Input: part model. Units: mm. Frame: model coordinates. Round coordinates to 2 decimals unless told otherwise and drop trailing zeros. Order: outer loops, then holes, each group sorted by start corner. A loop starts at its lowest first (then second) coordinate and runs counter-clockwise, first axis right, second up. Notation, with made-up numbers: (18.5, 57.25) - (29.5, 57.25) arc R32 ccw to (29.5, 95.25) - close; hole circle Ø1 at (26.5, 3). An arc over 180 degrees is marked (long way). One line per item, written item: value. Start each with the question number.
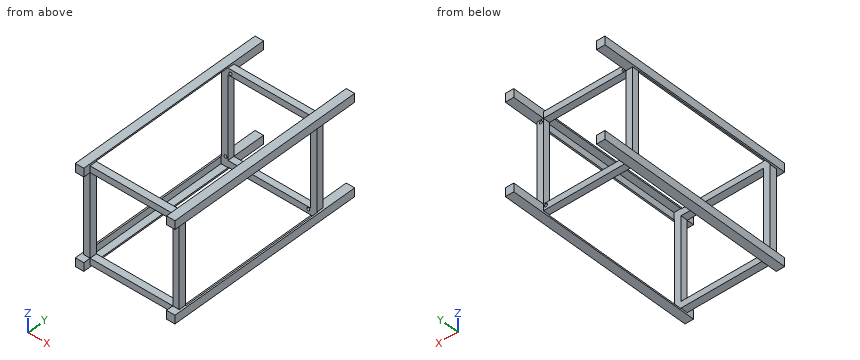
from build123d import *

# Parameters (mm, degrees)
SKETCH1_W           = 100
SKETCH1_H           = 100
BOSS_EXTRUDE1_DEPTH = 200
SKETCH2_W           = 83
SKETCH2_H           = 83
CUT_EXTRUDE1_DEPTH  = 200
SKETCH3_W           = 83
SKETCH3_H           = 14
SKETCH3_H_2         = 146.5
SKETCH3_H_3         = 66
CUT_EXTRUDE2_DEPTH  = 200
SKETCH4_W           = 83
SKETCH4_H           = 14
SKETCH4_H_2         = 146.5
SKETCH4_H_3         = 66
CUT_EXTRUDE3_DEPTH  = 200
SKETCH5_W           = 83
SKETCH5_H           = 4
SKETCH5_W_2         = 4
SKETCH5_H_2         = 83
CUT_EXTRUDE4_DEPTH  = 200
SKETCH8_W           = 97
SKETCH8_H           = 97
CUT_EXTRUDE5_DEPTH  = 146.5
CUT_EXTRUDE6_REACH  = 220.836
SKETCH9_R           = 1.5


with BuildPart() as part:
    # Sketch1 → Boss-Extrude1 (new body)
    with BuildSketch(Plane(origin=(0, 0, 0), x_dir=(1, 0, 0), z_dir=(0, 1, 0))):
        with Locations((50, 50)):
            Rectangle(SKETCH1_W, SKETCH1_H)
    extrude(amount=BOSS_EXTRUDE1_DEPTH)

    # Sketch2 → Cut-Extrude1 (cut)
    with BuildSketch(Plane(origin=(0, 200, 0), x_dir=(1, 0, 0), z_dir=(0, 1, 0))):
        with Locations((50, 50)):
            Rectangle(SKETCH2_W, SKETCH2_H)
    extrude(amount=-CUT_EXTRUDE1_DEPTH, mode=Mode.SUBTRACT)

    # Sketch3 → Cut-Extrude2 (cut)
    with BuildSketch(Plane.XY):
        with Locations((50, 0)):
            Rectangle(SKETCH3_W, SKETCH3_H)
        with Locations((50, 87.25)):
            Rectangle(SKETCH3_W, SKETCH3_H_2)
        with Locations((50, 200)):
            Rectangle(SKETCH3_W, SKETCH3_H_3)
    extrude(amount=-CUT_EXTRUDE2_DEPTH, mode=Mode.SUBTRACT)

    # Sketch4 → Cut-Extrude3 (cut)
    with BuildSketch(Plane.ZY):
        with Locations((-50, 0)):
            Rectangle(SKETCH4_W, SKETCH4_H)
        with Locations((-50, 87.25)):
            Rectangle(SKETCH4_W, SKETCH4_H_2)
        with Locations((-50, 200)):
            Rectangle(SKETCH4_W, SKETCH4_H_3)
    extrude(amount=-CUT_EXTRUDE3_DEPTH, mode=Mode.SUBTRACT)

    # Sketch5 → Cut-Extrude4 (cut)
    with BuildSketch(Plane.XZ.offset(-7)):
        with Locations((50, 0)):
            Rectangle(SKETCH5_W, SKETCH5_H)
        with Locations((100, -50)):
            Rectangle(SKETCH5_W_2, SKETCH5_H_2)
        with Locations((50, -100)):
            Rectangle(SKETCH5_W, SKETCH5_H)
        with Locations((0, -50)):
            Rectangle(SKETCH5_W_2, SKETCH5_H_2)
    extrude(amount=-CUT_EXTRUDE4_DEPTH, mode=Mode.SUBTRACT)

    # Sketch8 → Cut-Extrude5 (cut)
    with BuildSketch(Plane.XZ.offset(-160.5)):
        with Locations((50, -50)):
            Rectangle(SKETCH8_W, SKETCH8_H)
    extrude(amount=CUT_EXTRUDE5_DEPTH, mode=Mode.SUBTRACT)

    # Sketch9 → Cut-Extrude6 (cut, up to next)
    with BuildSketch(Plane(origin=(0, 167, 0), x_dir=(1, 0, 0), z_dir=(0, 1, 0)), mode=Mode.PRIVATE) as cut_extrude6_sk1:
        with Locations(Location((6, 89, 0), (0, 0, 270))):
            Circle(SKETCH9_R)
    cut_extrude6_tool1 = extrude(cut_extrude6_sk1.sketch, amount=-CUT_EXTRUDE6_REACH, mode=Mode.PRIVATE) & part.part
    # Sketch9 → Cut-Extrude6 (cut, up to next)
    with BuildSketch(Plane(origin=(0, 167, 0), x_dir=(1, 0, 0), z_dir=(0, 1, 0)), mode=Mode.PRIVATE) as cut_extrude6_sk2:
        with Locations(Location((89, 94, 0), (0, 0, 270))):
            Circle(SKETCH9_R)
    cut_extrude6_tool2 = extrude(cut_extrude6_sk2.sketch, amount=-CUT_EXTRUDE6_REACH, mode=Mode.PRIVATE) & part.part
    # Sketch9 → Cut-Extrude6 (cut, up to next)
    with BuildSketch(Plane(origin=(0, 167, 0), x_dir=(1, 0, 0), z_dir=(0, 1, 0)), mode=Mode.PRIVATE) as cut_extrude6_sk3:
        with Locations(Location((94, 11, 0), (0, 0, 270))):
            Circle(SKETCH9_R)
    cut_extrude6_tool3 = extrude(cut_extrude6_sk3.sketch, amount=-CUT_EXTRUDE6_REACH, mode=Mode.PRIVATE) & part.part
    # Sketch9 → Cut-Extrude6 (cut, up to next)
    with BuildSketch(Plane(origin=(0, 167, 0), x_dir=(1, 0, 0), z_dir=(0, 1, 0)), mode=Mode.PRIVATE) as cut_extrude6_sk4:
        with Locations(Location((11, 6, 0), (0, 0, 270))):
            Circle(SKETCH9_R)
    cut_extrude6_tool4 = extrude(cut_extrude6_sk4.sketch, amount=-CUT_EXTRUDE6_REACH, mode=Mode.PRIVATE) & part.part
    add(cut_extrude6_tool1.solids().sort_by_distance((6, 167, -89))[0], mode=Mode.SUBTRACT)
    add(cut_extrude6_tool2.solids().sort_by_distance((89, 167, -94))[0], mode=Mode.SUBTRACT)
    add(cut_extrude6_tool3.solids().sort_by_distance((94, 167, -11))[0], mode=Mode.SUBTRACT)
    add(cut_extrude6_tool4.solids().sort_by_distance((11, 167, -6))[0], mode=Mode.SUBTRACT)


solid = part.part
1. Section B-B (z = -31). Return the cut outline in (x, y), then the cut area to 4 significant figures.
2. Section C-C (x = 65.5). Return the cut outline in (y, z), then the cut area to 4 significant figures.
3. Section A-A (y = 64). Return the cut outline in (x, z), then the cut area to 3 significant figures.
4. Line query: line 1 (X direction, y = 165, z = -11); line 2 (X direction, y = 165, z = -89); line 3 (X direction, y = 162, z = -6). Output: solid intervals per line, ascending. Write a range as from..to.
5. Pin query (flat end, axial travel): pin 1 (7.5 mm diameter, centred on x = 60, y = 10, fed in from +Z); pin 2 (3.5 mm diameter, centred on y = 9.5, z = -58, fed in from -X); pin 3 (5 mm diameter, centred on x = 94.5, z = -48, fed in from +Y). Return the tip coordinate at first contact, or that it passes through.
Solved:
1. outline: (2, 7) - (8.5, 7) - (8.5, 14) - (2, 14) - close; (2, 160.5) - (8.5, 160.5) - (8.5, 167) - (2, 167) - close; (91.5, 7) - (98, 7) - (98, 14) - (91.5, 14) - close; (91.5, 160.5) - (98, 160.5) - (98, 167) - (91.5, 167) - close
1. area: 175.5 mm²
2. outline: (7, -98) - (14, -98) - (14, -91.5) - (7, -91.5) - close; (7, -8.5) - (14, -8.5) - (14, -2) - (7, -2) - close; (160.5, -98) - (167, -98) - (167, -91.5) - (160.5, -91.5) - close; (160.5, -8.5) - (167, -8.5) - (167, -2) - (160.5, -2) - close
2. area: 175.5 mm²
3. outline: (0, -100) - (8.5, -100) - (8.5, -98.5) - (1.5, -98.5) - (1.5, -91.5) - (0, -91.5) - close; (0, -8.5) - (1.5, -8.5) - (1.5, -1.5) - (8.5, -1.5) - (8.5, 0) - (0, 0) - close; (91.5, -100) - (100, -100) - (100, -91.5) - (98.5, -91.5) - (98.5, -98.5) - (91.5, -98.5) - close; (91.5, -1.5) - (98.5, -1.5) - (98.5, -8.5) - (100, -8.5) - (100, 0) - (91.5, 0) - close
3. area: 93.0 mm²
4. line 1: x = 2..8.5, 91.5..92.5, 95.5..98
4. line 2: x = 2..4.5, 7.5..8.5, 91.5..98
4. line 3: x = 0..9.5, 12.5..100
5. pin 1: stops at z = -2
5. pin 2: stops at x = 2
5. pin 3: stops at y = 167
